Design review of the part built by this model. Coordinates are the model's own, in mm. Coordinates: 2 decimals unless noted, no trailing zeros. Loops run counter-clockwise (first coordinate to the right, second up) from the corner with the lowest first, then second, coordinate; pieces in that order, holes last. Notation, with made-up numbers: (84, -21) -> (109, -21) arc R19 ccw to (109, 14) -> close; hole circle Ø8 at (63, 62). An arc over 180 degrees is marked (long way). Answer as a JSON object with one key per item and string values.
```python
from build123d import *

# Parameters (mm, degrees)
F0_R          = 10.375
F0_R_2        = 8.875
F1_DEPTH      = 2
F1_DEPTH_BACK = 2
F2_SIZE       = 1
F4_START      = 9.775
F3_R          = 0.75
F4_DEPTH      = 15.225


with BuildPart() as f1:
    # F0 (on Front) → F1 (new body, two sides)
    with BuildSketch(Plane.XZ) as f1_sk:
        Circle(F0_R)
        Circle(F0_R_2, mode=Mode.SUBTRACT)
    extrude(amount=F1_DEPTH)
    extrude(f1_sk.sketch, amount=-F1_DEPTH_BACK)

    # F2
    f2_edges = [f1.edges().sort_by_distance(p)[0] for p in [
        (-8.875, -2, 0),
        (-8.875, 2, 0),
    ]]
    chamfer(f2_edges, length=F2_SIZE)

    # F3 (on Top) → F4 (cut)
    with BuildSketch(Plane.XY.offset(F4_START)):
        with BuildLine():
            Line((-1.5, -1), (1.5, -1))
            ThreePointArc((1.5, -1), (2.2071067812, -0.7071067812), (2.5, 0))
            ThreePointArc((2.5, 0), (2.2071067812, 0.7071067812), (1.5, 1))
            Line((1.5, 1), (-1.5, 1))
            ThreePointArc((-1.5, 1), (-2.2071067812, 0.7071067812), (-2.5, 0))
            ThreePointArc((-2.5, 0), (-2.2071067812, -0.7071067812), (-1.5, -1))
        make_face()
        Circle(F3_R, mode=Mode.SUBTRACT)
        Circle(F3_R)
    extrude(amount=F4_DEPTH, mode=Mode.SUBTRACT)


solid = f1.part
```
1) Add section D-D, the plane y = 1.55. Give the boundary of the cut face in (x, z) (3 decimals), and give its area (3 significant figures).
Completed:
{"outline": "circle Ø20.75 at (0, 0); hole circle Ø18.85 at (0, 0)", "area": "59.1 mm²"}
2) Wall thickness on probe 1 along Z at (x, y) = (0, 0) (3 decimals); probe 2 along Z at (x, y) = (4.75, -0.9); probe 3 along X at (y, z) = (1.4, 1.5): over which ranges is each line inside the solid? List them lowest first.
Completed:
{"probe 1": "-10.375 to -8.875, 8.875 to 9.775", "probe 2": "-9.22 to -7.5, 7.5 to 9.22", "probe 3": "-10.27 to -9.15, 9.15 to 10.27"}
3) The part is to be moulded in two halves that separate along Z. For faces 1 (the cylindrical face through (-2.25, -0.03, -10.13)), 2 (the cylindrical face through (-1.924, 0.014, -8.664)), 3 (the flat face through (0, 0, 9.775)), say which applies: pulls with the +Z half, pulls with the -Z half, needs draft (parallel to the pull), parting line crosses it, or undercut.
Completed:
{"face 1": "parting line crosses it", "face 2": "undercut", "face 3": "pulls with the +Z half"}
4) Add section A-A, the plane z = 0. Give the boundary of the cut face in (x, y) (3 decimals), and give its area (4 significant figures).
Completed:
{"outline": "(-10.375, -2) -> (-9.875, -2) -> (-8.875, -1) -> (-8.875, 1) -> (-9.875, 2) -> (-10.375, 2) -> close; (8.875, -1) -> (9.875, -2) -> (10.375, -2) -> (10.375, 2) -> (9.875, 2) -> (8.875, 1) -> close", "area": "10.00 mm²"}
5) Add section B-B, the plane x = 0. Give the boundary of the cut face in (y, z) (3 decimals).
Completed:
{"outline": "(-2, -10.375) -> (2, -10.375) -> (2, -9.875) -> (1, -8.875) -> (-1, -8.875) -> (-2, -9.875) -> close; (-2, 9.875) -> (-1, 8.875) -> (1, 8.875) -> (2, 9.875) -> (2, 10.375) -> (1, 10.375) -> (1, 9.775) -> (-1, 9.775) -> (-1, 10.375) -> (-2, 10.375) -> close"}
6) Clearance check with a flat-ended pin moving along its axis: pin 1 Ø1 at (x, y) = (-1, 0) entering from +Z (3 decimals). State where the tip first meets the part, or that it passes through.
Completed:
{"pin 1": "z = 9.775"}
7) Add section C-C, the plane y = 0.35. Give the boundary of the cut face in (x, z) (3 decimals), and give its area (3 significant figures).
Completed:
{"outline": "(-2.437, 9.775) -> (-2.437, 10.085) arc R10.375 ccw (long way) to (2.437, 10.085) -> (2.437, 9.775) -> close; hole circle Ø17.75 at (0, 0)", "area": "88.3 mm²"}
